Part model, mm, in its own coordinate system. A direction names the side the tool comes from. Give positions to 0.01 mm unless a question says otherwise; leave off trailing zeros. Order: outer loops, then holes, each group sorted by start corner. A loop starts at its lowest first (then second) coordinate and runs counter-clockwise, first axis right, second up. Notation, with made-up numbers: (-25.5, 16) - (17.5, 16) arc R12 ccw to (17.5, 32) - close; hole circle Ø3 at (73, 89). An arc over 180 degrees is marked (long way). Use one line per item in the form item = value. Start each with the question number.
1. Band-saw the part on B-B, the plane z = 0. List the corners of the cut face in (x, y) (3 decimals).
2. Pull direction Z, two halves, no side cores. Call faces 3 (the face through (-2.3, 0, -2.3)), 4 (the face through (5.12, 56.35, -8.03)), 5 (the face through (8.69, 109.72, -1.02)): +Z half, -Z half, draft (parallel to the pull), parting line (faces both ways), or undercut.
3. Band-saw the part on C-C, the plane y = 71. List the corners of the cut face in (x, z) (3 decimals).
4. Pin check, flat tips, straight feed: P1, Ø1.5, axis at y = 26.5, z = 1.5, coming from the -X side; P2, Ø3.5, axis at y = 108.12, z = 0, coming from the +X side; P3, Ø6, axis at y = 100, z = -6, coming from the -X side; P4, Ø1, axis at x = -4, y = 31.5, coming from the -Z side. Stop position of each tip, or through.
5. Drill centre lines: line 1 (Y direction, x = 8.9, z = 0); line 2 (Z direction, x = 0, y = 33.5) (3 decimals); line 3 (Z direction, x = 0, y = 3.25) (3 decimals). Where is each one in solid material? Low to high.
6. Tool access for faces 1 (the face through (-0.1, 6.35, 3.5)), 2 (the face through (-8.685, 98.934, 1.754)): list every direction of +Z, -Z, +X, -X, +Y, -Y with a clear straight run to the whole face (end or side of a thin tool).
7. Band-saw the part on D-D, the plane z = -4.5. List the corners of the cut face in (x, y), plus the area to 3 significant figures.
8. Band-saw the part on A-A, the plane x = 0. List the corners of the cut face in (y, z) (3 decimals).
from build123d import *

# Parameters (mm, degrees)
SKETCH1_R                 = 9.525
BOSS_EXTRUDE1_DEPTH       = 114.3
SKETCH2_R                 = 8.095601674
CUT_EXTRUDE1_DEPTH        = 1
CUT_EXTRUDE1_DEPTH_BACK   = 107.95
SKETCH4_R                 = 1.89865
CUT_EXTRUDE2_DEPTH        = 114.3
CIRPATTERN1_COUNT         = 4
CIRPATTERN1_ANGLE         = 180
LPATTERN1_COUNT           = 2
LPATTERN1_PITCH           = 8.4582
LPATTERN1_COPY_1_SKETCH_R = 1.89865
LPATTERN1_COPY_1_DEPTH    = 114.3
LPATTERN1_COPY_2_SKETCH_R = 1.89865
LPATTERN1_COPY_2_DEPTH    = 114.3
LPATTERN1_COPY_3_SKETCH_R = 1.89865
LPATTERN1_COPY_3_DEPTH    = 114.3
SKETCH5_R                 = 2.921
CUT_EXTRUDE3_DEPTH        = 114.3


with BuildPart() as part:
    # Sketch1 → Boss-Extrude1 (new body)
    with BuildSketch(Plane(origin=(0, 0, 0), x_dir=(1, 0, 0), z_dir=(0, 1, 0))):
        Circle(SKETCH1_R)
    extrude(amount=BOSS_EXTRUDE1_DEPTH)

    # Sketch2 → Cut-Extrude1 (cut, two sides)
    with BuildSketch(Plane(origin=(0, 114.3, 0), x_dir=(1, 0, 0), z_dir=(0, 1, 0))) as cut_extrude1_sk:
        Circle(SKETCH2_R)
    extrude(amount=CUT_EXTRUDE1_DEPTH, mode=Mode.SUBTRACT)
    extrude(cut_extrude1_sk.sketch, amount=-CUT_EXTRUDE1_DEPTH_BACK, mode=Mode.SUBTRACT)

    # Sketch4 → Cut-Extrude2 (cut)
    with BuildSketch(Plane(origin=(0, 0, 0), x_dir=(0, 0, -1), z_dir=(1, 0, 0))):
        with Locations((0, 108.119085448)):
            Circle(SKETCH4_R)
    cut_extrude2 = extrude(amount=CUT_EXTRUDE2_DEPTH, mode=Mode.SUBTRACT)

    # CirPattern1: Cut-Extrude2 ×4 about axis
    cirpattern1_axis = Axis((0, 114.3, 0), (0, -1, 0))
    for i in range(1, CIRPATTERN1_COUNT):
        add(cut_extrude2.rotate(cirpattern1_axis, i * CIRPATTERN1_ANGLE / (CIRPATTERN1_COUNT - 1)), mode=Mode.SUBTRACT)

    # LPattern1: Cut-Extrude2 ×2
    with Locations(*[(0, -i * LPATTERN1_PITCH, 0) for i in range(1, LPATTERN1_COUNT)]):
        add(cut_extrude2, mode=Mode.SUBTRACT)

    # LPattern1 copy 1 sketch → LPattern1 copy 1 (cut)
    with BuildSketch(Plane(origin=(0, -8.4582, 0), x_dir=(0.866025404, 0, -0.5), z_dir=(0.5, 0, 0.866025404))):
        with Locations((0, 108.119085448)):
            Circle(LPATTERN1_COPY_1_SKETCH_R)
    extrude(amount=LPATTERN1_COPY_1_DEPTH, mode=Mode.SUBTRACT)

    # LPattern1 copy 2 sketch → LPattern1 copy 2 (cut)
    with BuildSketch(Plane(origin=(0, -8.4582, 0), x_dir=(0.866025404, 0, 0.5), z_dir=(-0.5, 0, 0.866025404))):
        with Locations((0, 108.119085448)):
            Circle(LPATTERN1_COPY_2_SKETCH_R)
    extrude(amount=LPATTERN1_COPY_2_DEPTH, mode=Mode.SUBTRACT)

    # LPattern1 copy 3 sketch → LPattern1 copy 3 (cut)
    with BuildSketch(Plane(origin=(0, -8.4582, 0), x_dir=(0, 0, 1), z_dir=(-1, 0, 0))):
        with Locations((0, 108.119085448)):
            Circle(LPATTERN1_COPY_3_SKETCH_R)
    extrude(amount=LPATTERN1_COPY_3_DEPTH, mode=Mode.SUBTRACT)

    # Sketch5 → Cut-Extrude3 (cut)
    with BuildSketch(Plane.XZ):
        Circle(SKETCH5_R)
    extrude(amount=-CUT_EXTRUDE3_DEPTH, mode=Mode.SUBTRACT)


solid = part.part
From the geometry:
q1.outline = (-9.525, 0) - (-2.921, 0) - (-2.921, 6.35) - (-8.096, 6.35) - (-8.096, 97.762) - (-9.525, 97.762) - close; (-9.525, 101.56) - (-8.096, 101.56) - (-8.096, 106.22) - (-9.525, 106.22) - close; (-9.525, 110.018) - (-8.096, 110.018) - (-8.096, 114.3) - (-9.525, 114.3) - close; (2.921, 0) - (9.525, 0) - (9.525, 97.762) - (8.096, 97.762) - (8.096, 6.35) - (2.921, 6.35) - close; (8.096, 101.56) - (9.525, 101.56) - (9.525, 106.22) - (8.096, 106.22) - close; (8.096, 110.018) - (9.525, 110.018) - (9.525, 114.3) - (8.096, 114.3) - close
q2.face_3 = draft
q2.face_4 = parting line
q2.face_5 = undercut
q3.outline = circle Ø19.05 at (0, 0); hole circle Ø16.191 at (0, 0)
q4.P1 = -9.5
q4.P2 = through
q4.P3 = -9.04
q4.P4 = -8.86
q5.line_1 = 0 to 97.76, 101.56 to 106.22, 110.02 to 114.3
q5.line_2 = -9.525 to -8.096, 8.096 to 9.525
q5.line_3 = -9.525 to -2.921, 2.921 to 9.525
q6.face_1 = +Y
q6.face_2 = +X, -X
q7.outline = (-8.39, 0) - (8.39, 0) - (8.39, 114.3) - (6.73, 114.3) - (6.73, 6.35) - (-6.73, 6.35) - (-6.73, 114.3) - (-8.39, 114.3) - close
q7.area = 466 mm²
q8.outline = (0, -9.525) - (114.3, -9.525) - (114.3, -8.096) - (6.35, -8.096) - (6.35, -2.921) - (0, -2.921) - close; (0, 2.921) - (6.35, 2.921) - (6.35, 8.096) - (114.3, 8.096) - (114.3, 9.525) - (0, 9.525) - close
